Autodesk Inventor part; units mm, degrees
ref_plane "YZ Plane" through (0, 0, 0) normal (1, 0, 0) x (0, 1, 0)
ref_plane "XZ Plane" through (0, 0, 0) normal (0, 1, 0) x (-1, 0, 0)
ref_plane "XY Plane" through (0, 0, 0) normal (0, 0, 1) x (1, 0, 0)
sketch "Sketch1" plane through (0, 0, 0) normal (0, 0, 1) x (1, 0, 0)
  line L0 (-0.1956, -75.4616) -> (-110.1956, -75.4616)
  line L1 (-110.1956, -75.4616) -> (-110.1956, 34.5384)
  line L2 (-110.1956, 34.5384) -> (-0.1956, 34.5384)
  line L3 (-110.1956, 34.5384) -> (-108.1956, 34.5384) construction
  line L4 (-108.1956, 12.5384) -> (-104.1956, 12.5384)
  line L5 (-104.1956, 12.5384) -> (-104.1956, -3.4616)
  line L6 (-104.1956, -3.4616) -> (-108.1956, -3.4616)
  line L7 (-108.1956, -3.4616) -> (-108.1956, 12.5384)
  line L8 (-110.1956, 34.5384) -> (-110.1956, 32.5384) construction
  line L9 (-110.1956, -20.4616) -> (-0.1956, -20.4616) construction
  line L10 (-108.1956, -53.4616) -> (-104.1956, -53.4616)
  line L11 (-104.1956, -53.4616) -> (-104.1956, -37.4616)
  line L12 (-104.1956, -37.4616) -> (-108.1956, -37.4616)
  line L13 (-108.1956, -37.4616) -> (-108.1956, -53.4616)
  line L14 (-88.1956, -73.4616) -> (-72.1956, -73.4616)
  line L15 (-72.1956, -73.4616) -> (-72.1956, -69.4616)
  line L16 (-72.1956, -69.4616) -> (-88.1956, -69.4616)
  line L17 (-88.1956, -69.4616) -> (-88.1956, -73.4616)
  line L18 (-22.1956, -73.4616) -> (-38.1956, -73.4616)
  line L19 (-38.1956, -73.4616) -> (-38.1956, -69.4616)
  line L20 (-38.1956, -69.4616) -> (-22.1956, -69.4616)
  line L21 (-22.1956, -69.4616) -> (-22.1956, -73.4616)
  circle A0 centre (-55.1956, -71.4616) radius 1.75
  circle A1 centre (-106.1956, -20.4616) radius 1.75
  line L22 (-0.1956, 34.5384) -> (-0.1956, -75.4616)
  line L23 (-110.1956, 34.5384) -> (-100.1956, 34.5384)
  line L24 (-100.1956, 34.5384) -> (-100.1956, 24.5384)
  line L25 (-100.1956, 24.5384) -> (-110.1956, 24.5384)
  line L26 (-110.1956, 24.5384) -> (-110.1956, 34.5384)
  line L27 (-0.1956, -25.4616) -> (-10.1956, -25.4616)
  line L28 (-10.1956, -25.4616) -> (-10.1956, -15.4616)
  line L29 (-10.1956, -15.4616) -> (-0.1956, -15.4616)
  line L30 (-72.5638, 12.5384) -> (-68.5638, 12.5384)
  line L31 (-68.5638, 12.5384) -> (-68.5638, -53.4616)
  line L32 (-68.5638, -53.4616) -> (-72.5638, -53.4616)
  line L33 (-72.5638, -53.4616) -> (-72.5638, 12.5384)
  line L34 (-60.5638, 12.5384) -> (-60.5638, -53.4616)
  line L35 (-56.5638, 12.5384) -> (-56.5638, -53.4616)
  line L36 (-48.5638, 12.5384) -> (-48.5638, -53.4616)
  line L37 (-44.5638, 12.5384) -> (-44.5638, -53.4616)
  line L38 (-36.5638, 12.5384) -> (-36.5638, -53.4616)
  line L39 (-32.5638, 12.5384) -> (-32.5638, -53.4616)
  line L40 (-60.5638, -53.4616) -> (-56.5638, -53.4616)
  line L41 (-48.5638, -53.4616) -> (-44.5638, -53.4616)
  line L42 (-36.5638, -53.4616) -> (-32.5638, -53.4616)
  line L43 (-60.5638, 12.5384) -> (-56.5638, 12.5384)
  line L44 (-48.5638, 12.5384) -> (-44.5638, 12.5384)
  line L45 (-36.5638, 12.5384) -> (-32.5638, 12.5384)
  line L46 (-110.1956, -75.4616) -> (-100.1956, -75.4616)
  line L47 (-100.1956, -75.4616) -> (-100.1956, -65.4616)
  line L48 (-100.1956, -65.4616) -> (-110.1956, -65.4616)
  line L49 (-110.1956, -65.4616) -> (-110.1956, -75.4616)
  dimension "d5" = 110
  dimension "d6" = 110
  dimension "d7" = 2
  dimension "d8" = 22
  dimension "d10" = 4
  dimension "d11" = 16
  dimension "d12" = 2
  dimension "d20" = 3.5
  dimension "d21" = 10
  dimension "d22" = 10
  dimension "d25" = 10
  dimension "d26" = 4
  dimension "d30" = 4
  dimension "d33" = 4
  dimension "d34" = 4
  dimension "d35" = 4
  dimension "d37" = 10
  dimension "d38" = 10
extrude "Extrusion3" add sketch "Sketch1" along normal blind 3 contours L0 L47 L48 L1 L25 L24 L2 L22 L29 L28 L27
extrude "Extrusion4" add sketch "Sketch1" along normal blind 8 contours L0 L1 L48 L47 | L27 L28 L29 L22 | L1 L2 L24 L25
fillet "Fillet1" radius 3 1 edges at (-110.1956, 34.5384, 4)
fillet "Fillet2" radius 2 1 edges at (-110.1956, -75.4616, 4)
fillet "Fillet3" radius 2 16 edges at (-32.5638, 12.5384, 1.5) (-36.5638, 12.5384, 1.5) (-48.5638, 12.5384, 1.5) (-44.5638, 12.5384, 1.5) (-56.5638, 12.5384, 1.5) (-68.5638, 12.5384, 1.5) (-60.5638, 12.5384, 1.5) (-72.5638, 12.5384, 1.5) (-68.5638, -53.4616, 1.5) (-72.5638, -53.4616, 1.5) (-60.5638, -53.4616, 1.5) (-56.5638, -53.4616, 1.5) (-48.5638, -53.4616, 1.5) (-44.5638, -53.4616, 1.5) (-36.5638, -53.4616, 1.5) (-32.5638, -53.4616, 1.5)
properties part number "base_agitador"
Geometry check sheet. Reference: the model listing, model coordinates, mm. A direction names the side the tool comes from. Round coordinates to 2 decimals unless told otherwise and drop trailing zeros. Loops run counter-clockwise (first coordinate to the right, second up) from the corner with the lowest first, then second, coordinate; pieces in that order, holes last. Notation, with made-up numbers: M -30,9.5 L -12,9.5 A28 ccw -12,29.5 Z; hole C 14.5,-21 d9. An arc over 180 degrees is marked long. Return JSON: item names as keys, results as strings. Group by question number.
(1) Section check D-D, the plane x = -8. Enter the section's corners in (y, z), and give its area (3 significant figures).
(2) Mould release check, pull along Y, two halves, no side actions. Record for faces 5 (the face through (-22.196, -71, 1)), 6 (the face through (-5, -20, 8)), 7 (the face through (-65, -75.462, 2)): pulls with the +Y half, pulls with the -Y half, needs draft (parallel to the pull), parting line crosses it, or undercut.
(3) Section check B-B, the plane y = 6. Enter the section's corners in (x, z), and give its area (3 significant figures).
(4) Go/stop test with flat-tipped pins: pin 1 (1 mm diameter, centred on x = -88, y = -11, fed in from -Z); pin 2 (1.5 mm diameter, centred on x = -4.5, z = 6, fed in from +Y); pin 3 (6 mm diameter, centred on x = -40, y = -33, fed in from +Z); pin 4 (1 mm diameter, centred on y = 23, z = 6, fed in from -X). Record where each tip stops, or that it passes through.
(5) Section check C-C, the plane z = 4.5. Enter the section's corners in (x, y).
(6) Set-up check for faces 1 (the face through (-5, -15.462, 5)), 2 (the face through (-10.196, -21, 5)), 3 (the face through (-106, -37.462, 1)), 4 (the face through (-105, 24.538, 5)): record each of +Z, -Z, +X, -X, +Y, -Y from which the full face is reachable in a straight line by a thin tool's end or side.
(7) Scan lines: line 1 along X through (y, z) = (-35, 1); line 2 along X through (y, z) = (-44, 2.5); line 3 along Y through (x, z) = (-77, 2.75). Record each from-to range of solid material in increasing order. Write a range as [from, to].
(8) Section check A-A, the plane x = -30. Enter the section's corners in (y, z).
Data:
{
 "1": {"outline": "M -75.46,0 L 34.54,0 L 34.54,3 L -15.46,3 L -15.46,8 L -25.46,8 L -25.46,3 L -75.46,3 Z", "area": "380 mm²"},
 "2": {"face 5": "undercut", "face 6": "needs draft", "face 7": "pulls with the -Y half"},
 "3": {"outline": "M -110.2,0 L -108.2,0 L -108.2,3 L -110.2,3 Z; M -104.2,0 L -72.56,0 L -72.56,3 L -104.2,3 Z; M -68.56,0 L -60.56,0 L -60.56,3 L -68.56,3 Z; M -56.56,0 L -48.56,0 L -48.56,3 L -56.56,3 Z; M -44.56,0 L -36.56,0 L -36.56,3 L -44.56,3 Z; M -32.56,0 L -0.2,0 L -0.2,3 L -32.56,3 Z", "area": "270 mm²"},
 "4": {"pin 1": "z = 0", "pin 2": "y = -15.46", "pin 3": "z = 3", "pin 4": "through"},
 "5": {"outline": "M -110.2,-73.46 A2 ccw -108.2,-75.46 L -100.2,-75.46 L -100.2,-65.46 L -110.2,-65.46 Z; M -110.2,24.54 L -100.2,24.54 L -100.2,34.54 L -107.2,34.54 A3 ccw -110.2,31.54 Z; M -10.2,-25.46 L -0.2,-25.46 L -0.2,-15.46 L -10.2,-15.46 Z"},
 "6": {"face 1": "+Z, +X, -X, +Y", "face 2": "+Z, -X, +Y, -Y", "face 3": "+Z, -Z", "face 4": "+Z, +X, -X"},
 "7": {"line 1": "[-110.2, -72.56], [-68.56, -60.56], [-56.56, -48.56], [-44.56, -36.56], [-32.56, -0.2]", "line 2": "[-110.2, -108.2], [-104.2, -72.56], [-68.56, -60.56], [-56.56, -48.56], [-44.56, -36.56], [-32.56, -0.2]", "line 3": "[-75.46, -73.46], [-69.46, 34.54]"},
 "8": {"outline": "M -75.46,0 L -73.46,0 L -73.46,3 L -75.46,3 Z; M -69.46,0 L 34.54,0 L 34.54,3 L -69.46,3 Z"}
}
